Build history of the part. All positions in model axes, mm. A direction names the side the tool comes from. Round coordinates to 2 decimals unless told otherwise and drop trailing zeros. Order: outer loops, then holes, each group sorted by start corner. A loop starts at its lowest first (then second) coordinate and runs counter-clockwise, first axis right, second up. Notation, with made-up numbers: (18.25, -27) -> (27.25, -27) arc R17 cw to (27.25, -17) -> close; hole circle Ø2 at (23.25, 17). An arc over 180 degrees is marked (long way). Use a Markdown table: item, result. Add a question column.
Item 1: Slice it at C-C, the plane y = 50. Give the cut face in (x, z), plus the area to 3 significant figures.
Item 2: Slice it at B-B, the plane z = 1.5. Give the cut face in (x, y), plus the area to 3 significant figures.
Item 3: 3-axis set-ups, long thin cutter, end or side, ignore diameter. For faces 1 (the face through (-22.752, 49.824, 14.381)), 2 (the face through (-28, 50, 6)), 3 (the face through (-50, 43.75, 4)), 4 (the face through (-49.9, 46.75, 0.5)), 5 (the face through (-30.75, 57, 14)): which of +Z, -Z, +X, -X, +Y, -Y reach the whole face in a straight line?
Item 4: Slice it at A-A, the plane x = -45. Give the cut face in (y, z).
Item 5: Pin check, flat tips, straight feed: pin 1 (1 mm diameter, centred on y = 50.5, z = 14, fed in from +X); pin 2 (1.4 mm diameter, centred on y = 43.5, z = 12.5, fed in from -X); pin 3 (10 mm diameter, centred on x = -52.5, y = 54.5, fed in from +Z). Stop position of each tip, or through.
Item 6: Slice it at D-D, the plane x = -68. Give the cut face in (y, z), plus the area to 3 significant figures.
Item 7: Two-plate mould, pull along Y, no slides. Class faces 6 (the face through (-69.25, 50, 4)), 7 (the face through (-52, 40.5, 0.5)), 8 (the face through (-47, 54, 0)): released by +Y, released by -Y, zero draft, split by the parting line, or undercut.
Item 8: Probe L1, parallel to Y at x = -43, z = 4; L2, parallel to Z at x = -34, y = 51.5; L3, parallel to X at y = 44, z = 5.75. List the from-to ranges inside material, lowest first.
from build123d import *

# Parameters (mm, degrees)
PAD005_DEPTH    = 6
SKETCH015_W     = 38.5
SKETCH015_H     = 12.5
POCKET003_DEPTH = 5
SKETCH017_W     = 23.5
SKETCH017_H     = 7
POCKET010_DEPTH = 1
PAD006_DEPTH    = 17
POCKET011_DEPTH = 17
CHAMFER002_SIZE = 1
CHAMFER003_SIZE = 1
CHAMFER004_SIZE = 1


with BuildPart() as part:
    # Sketch016 → Pad005 (new body)
    with BuildSketch(Plane.XY):
        with BuildLine():
            Line((-23, 10), (-23, -10))
            Line((-23, -10), (19, -10))
            ThreePointArc((19, -10), (29, 0), (19, 10))
            Line((-23, 10), (19, 10))
        make_face()
    extrude(amount=PAD005_DEPTH)

    # Sketch015 (on Face6 of Pad005) → Pocket003 (cut)
    with BuildSketch(Plane.XY.offset(6)):
        Rectangle(SKETCH015_W, SKETCH015_H)
    extrude(amount=-POCKET003_DEPTH, mode=Mode.SUBTRACT)

    # Sketch017 (on Face11 of Pocket003) → Pocket010 (cut)
    with BuildSketch(Plane.XY.offset(1)):
        with Locations((0.25, 0.25)):
            Rectangle(SKETCH017_W, SKETCH017_H)
    extrude(amount=-POCKET010_DEPTH, mode=Mode.SUBTRACT)

    # Sketch018 (on Face5 of Pocket010) → Pad006 (join)
    with BuildSketch(Plane.XY.offset(6)):
        with BuildLine():
            Line((19.25, 8), (19.25, -8))
            ThreePointArc((19.25, -8), (27.25, 0), (19.25, 8))
        make_face()
    extrude(amount=PAD006_DEPTH)

    # Sketch019 (on Face16 of Pad006) → Pocket011 (cut)
    with BuildSketch(Plane.XY.offset(23)):
        with BuildLine():
            Line((19.25, -6.25), (19.25, 6.25))
            ThreePointArc((19.25, -6.25), (25.5, 0), (19.25, 6.25))
        make_face()
    extrude(amount=-POCKET011_DEPTH, mode=Mode.SUBTRACT)

    # Chamfer002
    chamfer002_edges = [part.edges().sort_by_distance(p)[0] for p in [
        (-2, -10, 0),
    ]]
    chamfer(chamfer002_edges, length=CHAMFER002_SIZE)

    # Chamfer003
    chamfer003_edges = [part.edges().sort_by_distance(p)[0] for p in [
        (-23, 0, 0),
    ]]
    chamfer(chamfer003_edges, length=CHAMFER003_SIZE)

    # Chamfer004
    chamfer004_edges = [part.edges().sort_by_distance(p)[0] for p in [
        (-23, 10, 3.5),
        (-23, -10, 3.5),
    ]]
    chamfer(chamfer004_edges, length=CHAMFER004_SIZE)


with BuildPart() as part_1:
    # Body006 placement: moved
    add(part.part.moved(Location((-50, 50, 0))))


solid = part_1.part
Check sheet entries:
| question | item | result |
|---|---|---|
| 1 | outline | (-73, 1) -> (-72, 0) -> (-61.5, 0) -> (-61.5, 1) -> (-69.25, 1) -> (-69.25, 6) -> (-73, 6) -> close; (-38, 0) -> (-22, 0) -> (-21, 1) -> (-21, 6) -> (-22.75, 6) -> (-22.75, 23) -> (-24.5, 23) -> (-24.5, 6) -> (-30.75, 6) -> (-30.75, 1) -> (-38, 1) -> close |
| 1 | area | 125 mm2 |
| 2 | outline | (-73, 41) -> (-72, 40) -> (-31, 40) arc R10 ccw to (-31, 60) -> (-72, 60) -> (-73, 59) -> close; hole (-69.25, 43.75) -> (-30.75, 43.75) -> (-30.75, 56.25) -> (-69.25, 56.25) -> close |
| 2 | area | 515 mm2 |
| 3 | face 1 | +Z, +X |
| 3 | face 2 | +Z, -X |
| 3 | face 3 | +Z |
| 3 | face 4 | +Z, -Z |
| 3 | face 5 | +Z, -X, +Y, -Y |
| 4 | outline | (40, 1) -> (41, 0) -> (46.75, 0) -> (46.75, 1) -> (43.75, 1) -> (43.75, 6) -> (40, 6) -> close; (53.75, 0) -> (59, 0) -> (60, 1) -> (60, 6) -> (56.25, 6) -> (56.25, 1) -> (53.75, 1) -> close |
| 5 | pin 1 | x = -22.75 |
| 5 | pin 2 | x = -30.75 |
| 5 | pin 3 | z = 6 |
| 6 | outline | (40, 1) -> (41, 0) -> (59, 0) -> (60, 1) -> (60, 6) -> (56.25, 6) -> (56.25, 1) -> (43.75, 1) -> (43.75, 6) -> (40, 6) -> close |
| 6 | area | 56.5 mm2 |
| 7 | face 6 | undercut |
| 7 | face 7 | released by -Y |
| 7 | face 8 | zero draft |
| 8 | L1 | 40 to 43.75, 56.25 to 60 |
| 8 | L2 | 0 to 1 |
| 8 | L3 | -73 to -69.25, -30.75 to -23 |
